```python
from build123d import *

# Parameters (mm, degrees)
SKETCH1_W           = 100
SKETCH1_H           = 135
BOSS_EXTRUDE1_DEPTH = 30
SKETCH2_W           = 98.5
SKETCH2_H           = 133.5
CUT_EXTRUDE1_DEPTH  = 28.5
FILLET21_R          = 2
FILLET22_R          = 2
CUT_EXTRUDE2_DEPTH  = 1.5


with BuildPart() as part:
    # Sketch1 → Boss-Extrude1 (new body)
    with BuildSketch(Plane.XY):
        Rectangle(SKETCH1_W, SKETCH1_H)
    extrude(amount=BOSS_EXTRUDE1_DEPTH)

    # Sketch2 → Cut-Extrude1 (cut)
    with BuildSketch(Plane.XY.offset(30)):
        Rectangle(SKETCH2_W, SKETCH2_H)
    extrude(amount=-CUT_EXTRUDE1_DEPTH, mode=Mode.SUBTRACT)

    # Fillet21
    fillet21_edges = [part.edges().sort_by_distance(p)[0] for p in [
        (50, -67.5, 15),
        (-50, -67.5, 15),
        (-50, 67.5, 15),
        (50, 67.5, 15),
    ]]
    fillet(fillet21_edges, radius=FILLET21_R)

    # Fillet22
    fillet22_edges = [part.edges().sort_by_distance(p)[0] for p in [
        (49.25, 66.75, 15.75),
        (49.25, -66.75, 15.75),
        (-49.25, -66.75, 15.75),
        (-49.25, 66.75, 15.75),
    ]]
    fillet(fillet22_edges, radius=FILLET22_R)

    # Sketch4 → Cut-Extrude2 (cut)
    with BuildSketch(Plane.XZ.offset(67.5)):
        Polygon((0, 10), (0, 7.5), (7.5, 7.5), (7.5, 12.5), (0, 12.5), align=None)
        Polygon((-7.5, 7.5), (0, 7.5), (0, 10), (0, 12.5), (-7.5, 12.5), align=None)
    extrude(amount=-CUT_EXTRUDE2_DEPTH, mode=Mode.SUBTRACT)


solid = part.part
```
Model file for the job. Use its own axes, mm. A direction names the side the tool comes from. Give positions to 0.01 mm unless a question says otherwise; leave off trailing zeros. Loops run counter-clockwise (first coordinate to the right, second up) from the corner with the lowest first, then second, coordinate; pieces in that order, holes last. Notation, with made-up numbers: (36.5, -4.75) -> (81.5, -4.75) arc R25 ccw to (81.5, 32.25) -> close; hole circle Ø10 at (13, 89). An arc over 180 degrees is marked (long way). Use CSV: the item, a comma, the result in double quotes. Start each with the question number.
1) Tool access for faces 5 (the flat face through (-50, -1, 15)), 6 (the flat face through (-1, 1, 1.5)): list every direction of +Z, -Z, +X, -X, +Y, -Y with a clear straight run to the whole face (end or side of a thin tool).
2) Wall check: line 1 (X direction, y = 17.5, z = 3); line 2 (Y direction, x = 30, z = 6); line 3 (Z direction, x = 18, y = -5.5). Give the ranges that are in metal, low to high.
3) Mould opens along Y. For faces 1 (the flat face through (-1, 66.75, 16)), 2 (the flat face through (50, -1, 15)), 3 (the flat face through (-1, 67.5, 15)), 4 (the flat face through (-1, -67.5, 15)) say: released by +Y, released by -Y, zero draft, split by the parting line, or undercut.
4) Slice it at D-D on y = 5.5. Give the cut face in (x, z).
5) Slice it at B-B on z = 4.5. Give the cut face in (x, y).
6) Slice it at C-C on x = 34. Give the cut face in (y, z), plus the area to 3 significant figures.
7) Flat gauge pins, fed straight in: pin 1 Ø12 at (x, y) = (-14.5, 49) entering from +Z; pin 2 Ø0.6 at (y, z) = (-67, 10.5) entering from -X. Where does each tip first touch, or does it go through?
8) Slice it at A-A on x = -1.5. Give the cut face in (y, z).
Computed values:
1,face 5,"+Z, -Z, -X, +Y, -Y"
1,face 6,"+Z"
2,line 1,"x = -50 to -49.25, 49.25 to 50"
2,line 2,"y = -67.5 to -66.75, 66.75 to 67.5"
2,line 3,"z = 0 to 1.5"
3,face 1,"undercut"
3,face 2,"zero draft"
3,face 3,"released by +Y"
3,face 4,"released by -Y"
4,outline,"(-50, 0) -> (50, 0) -> (50, 30) -> (49.25, 30) -> (49.25, 1.5) -> (-49.25, 1.5) -> (-49.25, 30) -> (-50, 30) -> close"
5,outline,"(-50, -65.5) arc R2 ccw to (-48, -67.5) -> (48, -67.5) arc R2 ccw to (50, -65.5) -> (50, 65.5) arc R2 ccw to (48, 67.5) -> (-48, 67.5) arc R2 ccw to (-50, 65.5) -> close; hole (-49.25, -64.75) arc R2 ccw to (-47.25, -66.75) -> (47.25, -66.75) arc R2 ccw to (49.25, -64.75) -> (49.25, 64.75) arc R2 ccw to (47.25, 66.75) -> (-47.25, 66.75) arc R2 ccw to (-49.25, 64.75) -> close"
6,outline,"(-67.5, 0) -> (67.5, 0) -> (67.5, 30) -> (66.75, 30) -> (66.75, 1.5) -> (-66.75, 1.5) -> (-66.75, 30) -> (-67.5, 30) -> close"
6,area,"245 mm^2"
7,pin 1,"stops at z = 1.5"
7,pin 2,"stops at x = -49.6"
8,outline,"(-67.5, 0) -> (67.5, 0) -> (67.5, 30) -> (66.75, 30) -> (66.75, 1.5) -> (-66.75, 1.5) -> (-66.75, 7.5) -> (-67.5, 7.5) -> close; (-67.5, 12.5) -> (-66.75, 12.5) -> (-66.75, 30) -> (-67.5, 30) -> close"
